Model file for the job. Use its own axes, mm. A direction names the side the tool comes from. Coordinates: 2 decimals unless noted, no trailing zeros. Loops run counter-clockwise (first coordinate to the right, second up) from the corner with the lowest first, then second, coordinate; pieces in that order, holes last.
from build123d import *
from build123d.topology import SkipClean

# Parameters (mm, degrees)
SKETCH_1_W               = 20
SKETCH_1_H               = 44
SKETCH_1_R               = 4.2
EXTRUDE_1_DEPTH          = 7
SKETCH_2_W               = 20
SKETCH_2_H               = 44
EXTRUDE_2_DEPTH          = 3
SKETCH_3_W               = 20
SKETCH_3_H               = 26
SKETCH_3_R               = 3
EXTRUDE_4_DEPTH          = 8
EXTRUDE_5_DEPTH          = 4
EXTRUDE_6_DEPTH          = 4
CHAMFER_1_SIZE           = 2
FILLET_2_R               = 5
FILLET_3_R               = 1
FILLET_4_R               = 2
SKETCH_6_W               = 16
SKETCH_6_H               = 37
EXTRUDE_7_DEPTH          = 10
EXTRUDE_START            = 7
SKETCH_7_R               = 4.2
EXTRUDE_8_DEPTH          = 7
CHAMFER_2_SIZE           = 2
SKETCH_8_W               = 20
SKETCH_8_H               = 44
EXTRUDE_9_DEPTH          = 3
SKETCH_9_W               = 20
SKETCH_9_H               = 26
SKETCH_9_R               = 3
EXTRUDE_10_DEPTH         = 8
EXTRUDE_11_DEPTH         = 4
EXTRUDE_12_DEPTH         = 4
FILLET_5_R               = 2
FILLET_7_R               = 1
FILLET_8_R               = 5
SKETCH_12_W              = 3
SKETCH_12_H              = 4
CUT_EXTRUDE_1_DEPTH      = 88.549985722
EXTRUDE_13_DEPTH         = 4
EXTRUDE_14_DEPTH         = 4
CUT_EXTRUDE_2_DEPTH      = 86.819578186
CUT_EXTRUDE_2_DEPTH_BACK = 86.819578186
SKETCH_15_R              = 4.2
SKETCH_16_R              = 6
SKETCH_16_R_2            = 4.2
EXTRUDE_15_DEPTH         = 1
EXTRUDE_START_2          = 1
SKETCH_17_R              = 6
SKETCH_17_R_2            = 4.2
EXTRUDE_16_DEPTH         = 1
CHAMFER_3_SIZE           = 2
FILLET_9_R               = 4


with BuildPart() as part:
    # Эскиз1 → Бобышка-Вытянуть1 (new body)
    with BuildSketch(Plane.XY):
        with Locations((0, 22)):
            Rectangle(SKETCH_1_W, SKETCH_1_H)
        with Locations((0, 32)):
            Circle(SKETCH_1_R, mode=Mode.SUBTRACT)
    extrude(amount=EXTRUDE_1_DEPTH)

    # Эскиз2 → Бобышка-Вытянуть2 (add)
    with BuildSketch(Plane.XY.offset(7)):
        with Locations((0, 22)):
            Rectangle(SKETCH_2_W, SKETCH_2_H)
    extrude(amount=EXTRUDE_2_DEPTH)

    # Эскиз3 → Бобышка-Вытянуть4 (add)
    with BuildSketch(Plane(origin=(0, 0, 0), x_dir=(1, 0, 0), z_dir=(0, 1, 0))):
        with Locations((0, -23)):
            Rectangle(SKETCH_3_W, SKETCH_3_H)
        with Locations(Location((0, -26, 0), (0, 0, 270))):
            Circle(SKETCH_3_R, mode=Mode.SUBTRACT)
    extrude(amount=EXTRUDE_4_DEPTH)

    # Эскиз4 → Бобышка-Вытянуть5 (add)
    with BuildSketch(Plane.ZY.offset(10)):
        Polygon((36, 8), (10, 8), (10, 23), align=None)
    extrude(amount=-EXTRUDE_5_DEPTH)

    # Эскиз5 → Бобышка-Вытянуть6 (add)
    with BuildSketch(Plane(origin=(10, 0, 0), x_dir=(0, 0, -1), z_dir=(1, 0, 0))):
        Polygon((-36, 8), (-10, 23), (-10, 8), align=None)
    extrude(amount=-EXTRUDE_6_DEPTH)

    # Фаска1
    chamfer_1_edges = [part.edges().sort_by_distance(p)[0] for p in [
        (10, 22, 0),
        (-10, 22, 0),
    ]]
    chamfer(chamfer_1_edges, length=CHAMFER_1_SIZE)

    # Скругление2
    fillet_2_edges = [part.edges().sort_by_distance(p)[0] for p in [
        (-10, 44, 6),
        (10, 44, 6),
    ]]
    fillet(fillet_2_edges, radius=FILLET_2_R)

    # Скругление3
    fillet_3_edges = [part.edges().sort_by_distance(p)[0] for p in [
        (10, 4, 36),
    ]]
    fillet(fillet_3_edges, radius=FILLET_3_R)

    # Скругление4
    fillet_4_edges = [part.edges().sort_by_distance(p)[0] for p in [
        (-8, 23, 10),
        (8, 23, 10),
    ]]
    fillet(fillet_4_edges, radius=FILLET_4_R)

    # Эскиз6 → Бобышка-Вытянуть7 (add)
    with BuildSketch(Plane(origin=(0, 0, 0), x_dir=(1, 0, 0), z_dir=(0, 1, 0))):
        with Locations((0, 18.5)):
            Rectangle(SKETCH_6_W, SKETCH_6_H)
    extrude(amount=EXTRUDE_7_DEPTH)

    # Эскиз7 → Бобышка-Вытянуть8 (add)
    with BuildSketch(Plane(origin=(0, 0, -37), x_dir=(-1, 0, 0), z_dir=(0, 0, -1)).offset(EXTRUDE_START)):
        Polygon((0, 0), (-10, 0), (-10, 44), (10, 44), (10, 0), align=None)
        with Locations(Location((0, 32, 0), (0, 0, 180))):
            Circle(SKETCH_7_R, mode=Mode.SUBTRACT)
    extrude(amount=-EXTRUDE_8_DEPTH)

    # Фаска2
    chamfer_2_edges = [part.edges().sort_by_distance(p)[0] for p in [
        (10, 22, -37),
        (-10, 22, -37),
    ]]
    chamfer(chamfer_2_edges, length=CHAMFER_2_SIZE)

    # Эскиз8 → Бобышка-Вытянуть9 (add)
    with BuildSketch(Plane(origin=(0, 0, -44), x_dir=(-1, 0, 0), z_dir=(0, 0, -1))):
        with Locations((0, 22)):
            Rectangle(SKETCH_8_W, SKETCH_8_H)
    extrude(amount=EXTRUDE_9_DEPTH)

    # Эскиз9 → Бобышка-Вытянуть10 (add)
    with BuildSketch(Plane(origin=(0, 0, 0), x_dir=(1, 0, 0), z_dir=(0, 1, 0))):
        with Locations((0, 60)):
            Rectangle(SKETCH_9_W, SKETCH_9_H)
        with Locations(Location((0, 64, 0), (0, 0, 270))):
            Circle(SKETCH_9_R, mode=Mode.SUBTRACT)
    extrude(amount=EXTRUDE_10_DEPTH)

    # Эскиз10 → Бобышка-Вытянуть11 (add)
    with BuildSketch(Plane.ZY.offset(10)):
        Polygon((-73, 8), (-47, 8), (-47, 22), align=None)
    extrude(amount=-EXTRUDE_11_DEPTH)

    # Эскиз11 → Бобышка-Вытянуть12 (add)
    with BuildSketch(Plane(origin=(10, 0, 0), x_dir=(0, 0, -1), z_dir=(1, 0, 0))):
        Polygon((47, 8), (47, 22), (73, 8), align=None)
    extrude(amount=-EXTRUDE_12_DEPTH)

    # Скругление5
    fillet_5_edges = [part.edges().sort_by_distance(p)[0] for p in [
        (-8, 22, -47),
        (8, 22, -47),
    ]]
    fillet(fillet_5_edges, radius=FILLET_5_R)

    # Скругление7
    fillet_7_edges = [part.edges().sort_by_distance(p)[0] for p in [
        (10, 4, -73),
    ]]
    fillet(fillet_7_edges, radius=FILLET_7_R)

    # Скругление8
    fillet_8_edges = [part.edges().sort_by_distance(p)[0] for p in [
        (-10, 44, -43),
        (10, 44, -43),
    ]]
    fillet(fillet_8_edges, radius=FILLET_8_R)

    # Эскиз12 → Вырез-Вытянуть1 (cut, through all)
    with BuildSketch(Plane(origin=(10, 0, 0), x_dir=(0, 0, -1), z_dir=(1, 0, 0))):
        with Locations((-5.5, 32)):
            Rectangle(SKETCH_12_W, SKETCH_12_H)
        with Locations((42.5, 32)):
            Rectangle(SKETCH_12_W, SKETCH_12_H)
    extrude(amount=-CUT_EXTRUDE_1_DEPTH, mode=Mode.SUBTRACT)

    # Эскиз13 → Бобышка-Вытянуть13 (add)
    with BuildSketch(Plane(origin=(8, 0, 0), x_dir=(0, 0, -1), z_dir=(1, 0, 0))):
        Polygon((0, 10), (18.5, 10), (0, 20), align=None)
        Polygon((37, 10), (37, 20), (18.5, 10), align=None)
    extrude(amount=-EXTRUDE_13_DEPTH)

    # Эскиз14 → Бобышка-Вытянуть14 (add)
    with BuildSketch(Plane.ZY.offset(8)):
        Polygon((0, 10), (-18.5, 10), (0, 20), align=None)
        Polygon((-37, 10), (-37, 20), (-18.5, 10), align=None)
    extrude(amount=-EXTRUDE_14_DEPTH)

    # Эскиз15 → Вырез-Вытянуть2 (cut, two sides: drawn at the far end of the back side and taken through both)
    with SkipClean():  # the faces are left unmerged after this step: merging them gives an invalid solid
        with BuildSketch(Plane(origin=(0, 0, -37), x_dir=(-1, 0, 0), z_dir=(0, 0, -1)).offset(-CUT_EXTRUDE_2_DEPTH_BACK)):
            with Locations((0, 32)):
                Circle(SKETCH_15_R)
        extrude(amount=CUT_EXTRUDE_2_DEPTH + CUT_EXTRUDE_2_DEPTH_BACK, mode=Mode.SUBTRACT)

    # Эскиз16 → Бобышка-Вытянуть15 (add)
    with SkipClean():  # the faces are left unmerged after this step: merging them gives an invalid solid
        with BuildSketch(Plane(origin=(0, 0, -37), x_dir=(-1, 0, 0), z_dir=(0, 0, -1))):
            with Locations((0, 32)):
                Circle(SKETCH_16_R)
            with Locations((0, 32)):
                Circle(SKETCH_16_R_2, mode=Mode.SUBTRACT)
        extrude(amount=-EXTRUDE_15_DEPTH)

    # Эскиз17 → Бобышка-Вытянуть16 (add)
    with SkipClean():  # the faces are left unmerged after this step: merging them gives an invalid solid
        with BuildSketch(Plane(origin=(0, 0, 0), x_dir=(-1, 0, 0), z_dir=(0, 0, -1)).offset(EXTRUDE_START_2)):
            with Locations((0, 32)):
                Circle(SKETCH_17_R)
            with Locations((0, 32)):
                Circle(SKETCH_17_R_2, mode=Mode.SUBTRACT)
        extrude(amount=-EXTRUDE_16_DEPTH)

    # Фаска3
    chamfer_3_edges = [part.edges().sort_by_distance(p)[0] for p in [
        (0, 8, -73),
        (0, 8, 36),
    ]]
    chamfer(chamfer_3_edges, length=CHAMFER_3_SIZE)

    # Скругление9
    fillet_9_edges = [part.edges().sort_by_distance(p)[0] for p in [
        (-10, 4, 36),
        (-10, 4, -73),
    ]]
    fillet(fillet_9_edges, radius=FILLET_9_R)


solid = part.part
Q1. Mould opens along Z. For faces 5 (the cylindrical face through (-8, 43, -42)), 6 (the flat face through (1, 3, 36)), 7 (the flat face through (6.03, 15.07, -27.88)) say: +Z half, -Z half, draft (parallel to the pull), parting line (faces both ways), or undercut.
Answers:
face 5: draft
face 6: +Z half
face 7: undercut
Q2. Which spindle directions (+Z, -Z, +X, -X, +Y, -Y) get a long thin tool onto all of the face, cutting with end or side? Do faces 1 (the flat face through (-9, 22, -38)), 2 (the cylindrical face through (1.301, 26.143, -0.507)), 3 (the flat face through (-7, 32, 7)), 4 (the flat face through (0, 0, -19)). Say none if no direction does.
Answers:
face 1: -X, +Y, -Y
face 2: none
face 3: +X, -X
face 4: +Z, -Z, +X, -X, -Y
Q3. Slice it at D-D (x = 7). List the corners of the cut face in (y, z), and give its area (3 significant figures).
Answers:
outline: (0, -73) - (8, -73) - (21.43, -48.05) arc R2 cw to (23.19, -47) - (43.58, -47) - (43.58, -37) - (20, -37) - (10, -18.5) - (20, 0) - (43.58, 0) - (43.58, 10) - (24.16, 10) arc R2 cw to (22.42, 11) - (8, 36) - (0, 36) - close; hole (30, -44) - (34, -44) - (34, -41) - (30, -41) - close; hole (30, 4) - (34, 4) - (34, 7) - (30, 7) - close
area: 2,200 mm2
Q4. Flat gauge pins, fed straight in: P1, Ø11, axis at x = 0, y = 32, coming from the -Z side; P2, Ø2, axis at y = 14.5, z = -35.5, coming from the +X side; P3, Ø1.2, axis at x = 7.5, y = 32.5, coming from the +Z side; P4, Ø3, axis at x = -4, z = 22, coming from the -Y side. Where does each tip first touch, or does it go through?
Answers:
P1: stops at z = -47
P2: stops at x = 8
P3: stops at z = 10
P4: stops at y = 0
Q5. Slice it at C-C (x = 0). Count the separate pieces of the cut face and the enclosed holes in it, and give its area (3 significant figures).
Answers:
separate pieces: 5
enclosed holes: 0
area: 1,410 mm2
Q6. Drill centre lines: line 1 (Y direction, x = 0, z = -36.15); line 2 (X direction, y = 14, z = -57); line 3 (X direction, y = 4, z = 26). Where is each one in solid material? Low to high.
Answers:
line 1: y = 0 to 10, 26 to 27.8, 36.2 to 38
line 2: x = -10 to -6, 6 to 10
line 3: x = -10 to -3, 3 to 10
Q7. Slice it at A-A (z = -64). List the corners of the cut face in (x, y).
Answers:
outline: (-10, 0) - (-3, 0) - (-3, 8) - (-6, 8) - (-6, 12.85) - (-10, 12.85) - close; (3, 0) - (10, 0) - (10, 12.85) - (6, 12.85) - (6, 8) - (3, 8) - close
